Input: part model. Units: mm. Frame: model coordinates. A direction names the side the tool comes from. Coordinates: 2 decimals unless noted, no trailing zeros. Write each loop counter-clockwise with the first axis right and the second up, starting at its lowest first coordinate (ties: lowest second). Pieces come first, ordered by that corner, then holes. Notation, with made-up numbers: (19.25, 10) - (26.25, 10) arc R15 ccw to (26.25, 30) - close; hole circle Ø3 at (9, 72.25). An arc over 180 degrees is marked (long way). Use a Markdown table: item, result. Add a question column.
Q1. Section query C-C (y = 5). Return the cut outline in (x, z).
Q2. Section query A-A (z = 0). Return the cut outline in (x, y), then the cut area to 3 significant figures.
Q3. Material intervals for probe 1 along Y at (x, z) = (0, 5.75); probe 2 along X at (y, z) = (11.5, 0); probe 3 along Y at (x, z) = (-4.25, -6.5), sorted ascending. Write a range as from..to.
Q4. Set-up query: faces 4 (the face through (6, 7.6, -2)), 5 (the face through (7.81, 15.44, 1.73)), 6 (the face through (1.464, 4.561, 4.614)). Return all of +Z, -Z, +X, -X, +Y, -Y with unobstructed straight access to the full face (end or side cutting, diameter ignored); none if empty.
Q5. Mould query, pull axis Z, two halves, no side actions, for faces 1 (the face through (7.1, 3.75, -3.69)), 2 (the face through (6, 14.9, 2)), 3 (the face through (-4.61, 4.69, -1.39)). Classes: released by +Z, released by -Z, zero draft, split by the parting line, or undercut.
Q6. Section query B-B (x = 0). Return the cut outline in (y, z), then the cut area to 3 significant figures.
Q7. Section query D-D (z = 2.25). Return the cut outline in (x, y).
Q8. Pin query (flat end, axial travel): P1, Ø5, axis at x = -6, y = 7, coming from the -Z side; P2, Ø5, axis at x = 4.5, y = 4, coming from the +Z side; P3, Ø1.5, axis at x = -1, y = 5.5, coming from the -Z side. Return the tip coordinate at first contact, or that it passes through.
from build123d import *

# Parameters (mm, degrees)
ESQUISSE4_W                  = 1.65
ESQUISSE4_H                  = 8
R_P_TITION_CIRCULAIRE1_COUNT = 2
R_P_TITION_CIRCULAIRE1_ANGLE = 90


with BuildPart() as part:
    # Esquisse2 → R_volution1 (revolve)
    with BuildSketch(Plane.XY, mode=Mode.PRIVATE) as r_volution1_sk:
        Polygon((2, 16), (8, 16), (8, 14.9), (6.11, 14.9), (6.11, 7.6), (8, 7.6), (8, 0), (2, 0), align=None)
    revolve(r_volution1_sk.sketch.rotate(Axis((0, 0, 0), (0, 1, 0)), 90), axis=Axis((0, 0, 0), (0, 1, 0)))

    # Esquisse4 → Trou pour taraudage pour trou taraud_ M4 (revolve, cut)
    with BuildSketch(Plane(origin=(0, 3.8, 0), x_dir=(0, 1, 0), z_dir=(1, 0, 0))):
        with Locations((0.825, 4)):
            Rectangle(ESQUISSE4_W, ESQUISSE4_H)
    trou_pour_taraudage_pour_trou_taraud_m4 = revolve(axis=Axis((0, 3.8, -6.35), (0, 0, 1)), mode=Mode.SUBTRACT)

    # R_p_tition circulaire1: Trou pour taraudage pour trou taraud_ M4 ×2 about axis
    r_p_tition_circulaire1_axis = Axis((0, 16, 0), (0, -1, 0))
    for i in range(1, R_P_TITION_CIRCULAIRE1_COUNT):
        add(trou_pour_taraudage_pour_trou_taraud_m4.rotate(r_p_tition_circulaire1_axis, i * R_P_TITION_CIRCULAIRE1_ANGLE / (R_P_TITION_CIRCULAIRE1_COUNT - 1)), mode=Mode.SUBTRACT)


solid = part.part
Values follow:
| question | item | result |
|---|---|---|
| 1 | outline | (-7.92, -1.13) arc R8 ccw (long way) to (1.13, 7.92) - (1.13, 1.65) arc R2 cw (long way) to (-1.65, -1.13) - close; (-7.92, 1.13) - (-1.65, 1.13) arc R2 cw to (-1.13, 1.65) - (-1.13, 7.92) arc R8 ccw to start |
| 2 | outline | (-8, 0) - (-2, 0) - (-2, 2.15) - (-8, 2.15) - close; (-8, 5.45) - (-2, 5.45) - (-2, 16) - (-8, 16) - (-8, 14.9) - (-6.11, 14.9) - (-6.11, 7.6) - (-8, 7.6) - close; (2, 0) - (8, 0) - (8, 7.6) - (6.11, 7.6) - (6.11, 14.9) - (8, 14.9) - (8, 16) - (2, 16) - close |
| 2 | area | 145 mm2 |
| 3 | probe 1 | 0..2.15, 5.45..16 |
| 3 | probe 2 | -6.11..-2, 2..6.11 |
| 3 | probe 3 | 0..7.6, 14.9..16 |
| 4 | face 4 | none |
| 4 | face 5 | +Y, -Y |
| 4 | face 6 | +Z |
| 5 | face 1 | split by the parting line |
| 5 | face 2 | zero draft |
| 5 | face 3 | undercut |
| 6 | outline | (0, -8) - (7.6, -8) - (7.6, -6.11) - (14.9, -6.11) - (14.9, -8) - (16, -8) - (16, -2) - (0, -2) - close; (0, 2) - (2.15, 2) - (2.15, 8) - (0, 8) - close; (5.45, 2) - (16, 2) - (16, 8) - (14.9, 8) - (14.9, 6.11) - (7.6, 6.11) - (7.6, 8) - (5.45, 8) - close |
| 6 | area | 145 mm2 |
| 7 | outline | (-7.68, 0) - (7.68, 0) - (7.68, 7.6) - (5.68, 7.6) - (5.68, 14.9) - (7.68, 14.9) - (7.68, 16) - (-7.68, 16) - (-7.68, 14.9) - (-5.68, 14.9) - (-5.68, 7.6) - (-7.68, 7.6) - close; hole circle Ø3.3 at (0, 3.8) |
| 8 | P1 | z = -7.19 |
| 8 | P2 | z = 7.75 |
| 8 | P3 | z = -8 |
